Design review of the part built by this model. Coordinates are the model's own, in mm. A direction names the side the tool comes from. Give positions to 0.01 mm unless a question says otherwise; leave off trailing zeros. Order: outer loops, then holes, each group sorted by start corner. A loop starts at its lowest first (then second) coordinate and runs counter-clockwise, first axis right, second up.
```python
from build123d import *

# Parameters (mm, degrees)
F1_W          = 110
F1_H          = 110
F1_R          = 1.25
F1_R_2        = 4
F2_DEPTH      = 55
F3_R          = 1.25
F3_R_2        = 4
F4_DEPTH      = 55.001
F4_DEPTH_BACK = 55.001
F5_R          = 1.25
F5_R_2        = 4
F6_DEPTH      = 42.3


with BuildPart() as f2:
    # F1 (on Top) → F2 (new body, symmetric)
    with BuildSketch(Plane.XY):
        Rectangle(F1_W, F1_H)
        with Locations((-15.5, -15.5)):
            Circle(F1_R, mode=Mode.SUBTRACT)
        with Locations((15.5, -15.5)):
            Circle(F1_R, mode=Mode.SUBTRACT)
        with Locations((-15.5, 15.5)):
            Circle(F1_R, mode=Mode.SUBTRACT)
        Circle(F1_R_2, mode=Mode.SUBTRACT)
        with Locations((15.5, 15.5)):
            Circle(F1_R, mode=Mode.SUBTRACT)
    extrude(amount=F2_DEPTH, both=True)

    # F3 (on Front) → F4 (cut, two sides)
    with BuildSketch(Plane.XZ) as f4_sk:
        with Locations((15.5, 15.5)):
            Circle(F3_R)
        Circle(F3_R_2)
        with Locations((-15.5, 15.5)):
            Circle(F3_R)
        with Locations((-15.5, -15.5)):
            Circle(F3_R)
        with Locations((15.5, -15.5)):
            Circle(F3_R)
    extrude(amount=-F4_DEPTH, mode=Mode.SUBTRACT)
    extrude(f4_sk.sketch, amount=F4_DEPTH_BACK, mode=Mode.SUBTRACT)

    # F5 (on Right) → F6 (cut, symmetric)
    with BuildSketch(Plane.YZ):
        with Locations((-15.5, 15.5)):
            Circle(F5_R)
        Circle(F5_R_2)
        with Locations((15.5, 15.5)):
            Circle(F5_R)
        with Locations((15.5, -15.5)):
            Circle(F5_R)
        with Locations((-15.5, -15.5)):
            Circle(F5_R)
    extrude(amount=F6_DEPTH, both=True, mode=Mode.SUBTRACT)


solid = f2.part
```
1. For line 1 along X through (y, z) = (-44.5, 15.5); line 2 along Y through (x, z) = (-23, 0), list the stretches that pass through material, from the lowest coordinate up.
Recorded:
line 1: x = -55 to -16.75, -14.25 to 14.25, 16.75 to 55
line 2: y = -55 to -4, 4 to 55
2. Take a section at A-A (z = 0). State the section outline as (x, y) points, then the cut area to 3 significant figures.
Recorded:
outline: (-55, -55) - (-4, -55) - (-4, -4) - (-42.3, -4) - (-42.3, 4) - (-4, 4) - (-4, 55) - (-55, 55) - close; (4, -55) - (55, -55) - (55, 55) - (4, 55) - (4, 4) - (42.3, 4) - (42.3, -4) - (4, -4) - close; hole circle Ø2.5 at (-15.5, -15.5); hole circle Ø2.5 at (-15.5, 15.5); hole circle Ø2.5 at (15.5, -15.5); hole circle Ø2.5 at (15.5, 15.5)
area: 10,600 mm2
3. For pin 1 (3 mm diameter, centred on x = -15.5, z = -15.5, fed in from -Y); pin 2 (5 mm diameter, centred on x = 0, z = 0, fed in from +Y), all flat-tipped, find the tip position at first contact; note any pin that passes through.
Recorded:
pin 1: stops at y = -55
pin 2: passes through
4. Machinability: for faces 4 (the face through (-22.288, -0.867, -3.905)), 5 (the face through (1.846, 28.549, -3.549)), which of the approach directions +Z, -Z, +X, -X, +Y, -Y give a long, thin tool a straight path to every point of the face, cutting with its end or side? Answer none if there is none.
Recorded:
face 4: none
face 5: +Y, -Y
5. Draft analysis for pull direction X (two halves, no side actions). For faces 1 (the face through (-1, 13, -55)), 2 (the face through (-55, -1, 1)), 3 (the face through (22.288, 1.846, -3.549)), state which applies: pulls with the +X half, pulls with the -X half, needs draft (parallel to the pull), parting line crosses it, or undercut.
Recorded:
face 1: needs draft
face 2: pulls with the -X half
face 3: undercut
